Could you check a few things on this model? Use its own coordinates, in mm. Face numbers are marked on the shaded views. Round coordinates to 2 decimals unless told otherwise and drop trailing zeros. Loops run counter-clockwise (first coordinate to the right, second up) from the corner with the lowest first, then second, coordinate; pieces in that order, holes last. Notation, with made-up numbers: M 50.5,19 L 100.5,19 A18 ccw 100.5,43 Z; hole C -24.75,-31.5 d9. An arc over 180 degrees is marked long. Return JSON: item names as keys, results as strings. Group by question number.
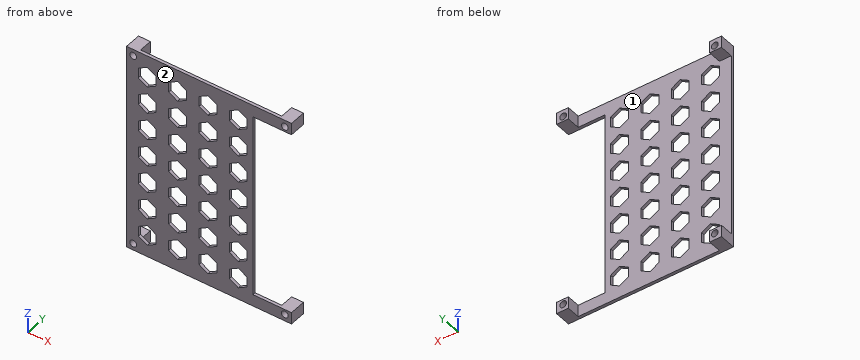
```python
from build123d import *

# Parameters (mm, degrees)
BOSS_EXTRUDE1_DEPTH  = 1
CUT_EXTRUDE1_DEPTH   = 1
LPATTERN1_COUNT      = 4
LPATTERN1_PITCH      = 10.266666667
LPATTERN1_COUNT_DIR2 = 7
LPATTERN1_PITCH_DIR2 = 9.311966128
SKETCH3_W            = 4
SKETCH3_H            = 4
BOSS_EXTRUDE2_DEPTH  = 4.5
SKETCH4_R            = 1.15
CUT_EXTRUDE2_DEPTH   = 5.5


with BuildPart() as part:
    # Sketch1 → Boss-Extrude1 (new body)
    with BuildSketch(Plane(origin=(0, 0, 0), x_dir=(1, 0, 0), z_dir=(0, 1, 0))):
        Polygon((0, 0), (55.8, 0), (55.8, 4), (42.8, 4), (42.8, 66.8), (55.8, 66.8), (55.8, 70.8), (0, 70.8), align=None)
    extrude(amount=BOSS_EXTRUDE1_DEPTH)

    # Sketch2 → Cut-Extrude1 (cut)
    with BuildSketch(Plane(origin=(0, 1, 0), x_dir=(1, 0, 0), z_dir=(0, 1, 0))):
        Polygon((7, 66.8), (4, 65.067949192), (4, 61.603847577), (7, 59.87179677), (10, 61.603847577), (10, 65.067949192), align=None)
    cut_extrude1 = extrude(amount=-CUT_EXTRUDE1_DEPTH, mode=Mode.SUBTRACT)

    # LPattern1: Cut-Extrude1 4 × 7
    with Locations(*[(i * LPATTERN1_PITCH, 0, j * LPATTERN1_PITCH_DIR2) for i in range(LPATTERN1_COUNT) for j in range(LPATTERN1_COUNT_DIR2) if (i, j) != (0, 0)]):
        add(cut_extrude1, mode=Mode.SUBTRACT)

    # Sketch3 → Boss-Extrude2 (add)
    with BuildSketch(Plane(origin=(0, 1, 0), x_dir=(1, 0, 0), z_dir=(0, 1, 0))):
        with Locations((2, 68.8)):
            Rectangle(SKETCH3_W, SKETCH3_H)
        with Locations((53.8, 68.8)):
            Rectangle(SKETCH3_W, SKETCH3_H)
        with Locations((53.8, 2)):
            Rectangle(SKETCH3_W, SKETCH3_H)
        with Locations((2, 2)):
            Rectangle(SKETCH3_W, SKETCH3_H)
    extrude(amount=BOSS_EXTRUDE2_DEPTH)

    # Sketch4 → Cut-Extrude2 (cut)
    with BuildSketch(Plane(origin=(0, 5.5, 0), x_dir=(1, 0, 0), z_dir=(0, 1, 0))):
        with Locations((2.25, 68.55)):
            Circle(SKETCH4_R)
        with Locations((53.55, 68.55)):
            Circle(SKETCH4_R)
    cut_extrude2 = extrude(amount=-CUT_EXTRUDE2_DEPTH, mode=Mode.SUBTRACT)

    # Mirror1: Cut-Extrude2 across plane
    add(cut_extrude2.mirror(Plane(origin=(0, 0, -35.4), x_dir=(1, 0, 0), z_dir=(0, 0, -1))), mode=Mode.SUBTRACT)


solid = part.part
```
1. If we section it at A-A, the plane x = 53.55: Please give me the cut outline in (y, z).
2. If we section it at B-B, the plane z = -2.25: Please give me the cut outline in (x, y).
3. If we section it at D-D, the plane x = 45: Please give me the cut outline in (y, z).
4. If we section it at C-C, the plane y = 2.95: Please give me the cut outline in (x, z).
5. I'm going to push flat-ended pins straight in: pin 1 Ø0.5 at (y, z) = (0.5, -25.5) entering from +X; pin 2 Ø2 at (x, z) = (27, -28.5) entering from +Y. Where does each tip first touch, or does it pass through?
6. I need wall thicknesses on probe 1 along Z at (x, y) = (53.55, 1.8); probe 2 along X at (y, z) = (2.3, -68.55); probe 3 along Z at (x, y) = (54, 4.25). Which ranges of each line are inside material? Lowest first, please.
7. We'd pull the mould along Z, two halves only. Please class the marked faces 1 and 2: +Z half, -Z half, draft (parallel to the pull), parting line (faces both ways), or undercut.
Geometry results:
{
 "1": {"outline": "M 0,-70.8 L 5.5,-70.8 L 5.5,-69.7 L 0,-69.7 Z; M 0,-67.4 L 5.5,-67.4 L 5.5,-66.8 L 0,-66.8 Z; M 0,-4 L 5.5,-4 L 5.5,-3.4 L 0,-3.4 Z; M 0,-1.1 L 5.5,-1.1 L 5.5,0 L 0,0 Z"},
 "2": {"outline": "M 0,0 L 1.1,0 L 1.1,5.5 L 0,5.5 Z; M 3.4,0 L 52.4,0 L 52.4,5.5 L 51.8,5.5 L 51.8,1 L 4,1 L 4,5.5 L 3.4,5.5 Z; M 54.7,0 L 55.8,0 L 55.8,5.5 L 54.7,5.5 Z"},
 "3": {"outline": "M 0,-70.8 L 1,-70.8 L 1,-66.8 L 0,-66.8 Z; M 0,-4 L 1,-4 L 1,0 L 0,0 Z"},
 "4": {"outline": "M 0,-70.8 L 4,-70.8 L 4,-66.8 L 0,-66.8 Z; M 0,-4 L 4,-4 L 4,0 L 0,0 Z; M 51.8,-70.8 L 55.8,-70.8 L 55.8,-66.8 L 51.8,-66.8 Z; M 51.8,-4 L 55.8,-4 L 55.8,0 L 51.8,0 Z; hole C 2.25,-68.55 d2.3; hole C 2.25,-2.25 d2.3; hole C 53.55,-68.55 d2.3; hole C 53.55,-2.25 d2.3"},
 "5": {"pin 1": "x = 42.8", "pin 2": "y = 1"},
 "6": {"probe 1": "-70.8 to -69.7, -67.4 to -66.8, -4 to -3.4, -1.1 to 0", "probe 2": "0 to 1.1, 3.4 to 4, 51.8 to 52.4, 54.7 to 55.8", "probe 3": "-70.8 to -69.61, -67.49 to -66.8, -4 to -3.31, -1.19 to 0"},
 "7": {"face 1": "undercut", "face 2": "draft"}
}
